Design review of the part built by this model. Coordinates are the model's own, in mm. A direction names the side the tool comes from. Give positions to 0.01 mm unless a question says otherwise; leave off trailing zeros. Loops run counter-clockwise (first coordinate to the right, second up) from the corner with the lowest first, then second, coordinate; pieces in that order, holes last. Notation, with made-up numbers: (76, 63.25) -> (90, 63.25) arc R27 ccw to (90, 102.25) -> close; hole circle Ø8 at (4, 84.25). An arc over 180 degrees is marked (long way). Use a Markdown table: item, result. Add a question column.
1. Add section A-A (z = 2). State the section outline as (x, y) points.
2. To check wall thickness, follow line 1 (X direction, y = 0, z = -3); line 2 (Z direction, x = 2, y = 1.75); line 3 (Z direction, x = 1, y = 2.25). State the ranges of each line that lie inside material, in increasing order.
3. For faces 1 (the flat face through (1.3, -1.3, 6)), 2 (the flat face through (0, 0, -10)), list the 3-axis set-ups (+Z, -Z, +X, -X, +Y, -Y) from which the entire face can be reached by the end or side of a thin tool; tool diameter is ignored.
4. For pin 1 Ø1.5 at (x, z) = (2, 3.5) entering from -Y, flat-tipped, find the tip position at first contact; note if it passes through.
Autodesk Inventor part; units mm, degrees
ref_plane "YZ Plane" through (0, 0, 0) normal (1, 0, 0) x (0, 1, 0)
ref_plane "XZ Plane" through (0, 0, 0) normal (0, 1, 0) x (-1, 0, 0)
ref_plane "XY Plane" through (0, 0, 0) normal (0, 0, 1) x (1, 0, 0)
sketch "スケッチ1" plane through (0, 0, 0) normal (0, 0, 1) x (1, 0, 0)
  circle A0 centre (0, 0) radius 1.5
  dimension "d0" = 3
extrude "押し出し1" add sketch "スケッチ1" along normal blind 6
sketch "スケッチ2" plane through (0, 0, 6) normal (0, 0, 1) x (1, 0, 0)
  circle A0 centre (0, 0) radius 1.5
  circle A1 centre (0, 0) radius 3
  dimension "d3" = 6
extrude "押し出し2" add sketch "スケッチ2" along normal blind 2 contours A0 | A1
fillet "フィレット1" radius 2 1 edges at (-3, 0, 8)
thread "ねじ1"
sketch "スケッチ3" plane through (0, 0, 0) normal (0, 0, -1) x (-1, 0, 0)
  circle A0 centre (0, 0) radius 1.5
extrude "押し出し3" add sketch "スケッチ3" along normal blind 9
sketch "スケッチ4" plane through (0, 0, -9) normal (0, 0, -1) x (-1, 0, 0)
  circle A0 centre (0, 0) radius 1.5
extrude "押し出し4" add sketch "スケッチ4" along normal blind 1
properties part number "SB　16mmなべネジ" material "Steel, Mild"
Taken from the geometry:
| question | item | result |
|---|---|---|
| 1 | outline | circle Ø3 at (0, 0) |
| 2 | line 1 | x = -1.5 to 1.5 |
| 2 | line 2 | z = 6 to 7.12 |
| 2 | line 3 | z = 6 to 7.36 |
| 3 | face 1 | -Z |
| 3 | face 2 | -Z, +X, -X, +Y, -Y |
| 4 | pin 1 | stops at y = -0.83 |
